Part model, mm, in its own coordinate system. A direction names the side the tool comes from. Round coordinates to 2 decimals unless told otherwise and drop trailing zeros. Write each loop counter-clockwise with the first axis right and the second up, starting at its lowest first coordinate (ties: lowest second). Pieces come first, ordered by that corner, then holes. Notation, with made-up numbers: M -9,23.25 L 2,23.25 A7 ccw 2,30.25 Z; hole C 37.25,-10 d3. An arc over 180 degrees is marked long. Answer as a JSON object with one key per item and string values. Group by question number.
1. Drop flat-ended pins along their axis: pin 1 (2 mm diameter, centred on x = 2.5, z = 1.5, fed in from -Y); pin 2 (1 mm diameter, centred on x = -7, z = 0.5, fed in from -Y); pin 3 (3 mm diameter, centred on y = 6, z = 0.5, fed in from -X). Give the stop position or say it passes through.
2. Band-saw the part on D-D, the plane x = -11.5. Write the cut outline in (y, z).
3. Band-saw the part on A-A, the plane y = 0. Write the cut outline in (x, z).
4. Two-plate mould, pull along X, no slides. Class faces 1 (the face through (-11.99, 0.53, -3.25)), 2 (the face through (-3.6, 14.3, -3.5)), 3 (the face through (-3.47, -15.62, 0.05)): +X half, -X half, draft (parallel to the pull), parting line (faces both ways), or undercut.
5. Band-saw the part on C-C, the plane z = -1.75. Write the cut outline in (x, y), plus the area to 3 significant figures.
6. Drill centre lines: line 1 (Y direction, x = 0, z = -3.15); line 2 (Y direction, x = 0, z = -1.25); line 3 (Z direction, x = -8.5, y = -11.5). Where is each one in solid material? Low to high. Write a range as from..to.
7. Which spindle directions (+Z, -Z, +X, -X, +Y, -Y) get a long thin tool onto all of the face, cutting with end or side? Do faces 4 (the face through (-11.99, 0.53, 3.25)), 5 (the face through (2, 12, -3)), 6 (the face through (-2.17, -9.76, -0.05)). Say none if no direction does.
from build123d import *

# Parameters (mm, degrees)
SKETCH_R      = 16
SKETCH_R_2    = 14.5
PAD_DEPTH     = 3.5
SKETCH001_R   = 14.5
SKETCH001_R_2 = 12
PAD001_DEPTH  = 3
SKETCH002_R   = 12
SKETCH002_R_2 = 10
PAD002_DEPTH  = 3.5


with BuildPart() as part:
    # Sketch → Pad (new body, symmetric)
    with BuildSketch(Plane.XY):
        Circle(SKETCH_R)
        Circle(SKETCH_R_2, mode=Mode.SUBTRACT)
    extrude(amount=PAD_DEPTH, both=True)

    # Sketch001 → Pad001 (join, symmetric)
    with BuildSketch(Plane.XY):
        Circle(SKETCH001_R)
        Circle(SKETCH001_R_2, mode=Mode.SUBTRACT)
    extrude(amount=PAD001_DEPTH, both=True)

    # Sketch002 → Pad002 (join, symmetric)
    with BuildSketch(Plane.XY):
        Circle(SKETCH002_R)
        Circle(SKETCH002_R_2, mode=Mode.SUBTRACT)
    extrude(amount=PAD002_DEPTH, both=True)


solid = part.part
Worked answers:
{
 "1": {"pin 1": "stops at y = -15.93", "pin 2": "stops at y = -14.62", "pin 3": "stops at x = -15.35"},
 "2": {"outline": "M -11.12,-3.5 L -8.83,-3.5 L -8.83,-3 L -3.43,-3 L -3.43,-3.5 L 3.43,-3.5 L 3.43,-3 L 8.83,-3 L 8.83,-3.5 L 11.12,-3.5 L 11.12,3.5 L 8.83,3.5 L 8.83,3 L 3.43,3 L 3.43,3.5 L -3.43,3.5 L -3.43,3 L -8.83,3 L -8.83,3.5 L -11.12,3.5 Z"},
 "3": {"outline": "M -16,-3.5 L -14.5,-3.5 L -14.5,-3 L -12,-3 L -12,-3.5 L -10,-3.5 L -10,3.5 L -12,3.5 L -12,3 L -14.5,3 L -14.5,3.5 L -16,3.5 Z; M 10,-3.5 L 12,-3.5 L 12,-3 L 14.5,-3 L 14.5,-3.5 L 16,-3.5 L 16,3.5 L 14.5,3.5 L 14.5,3 L 12,3 L 12,3.5 L 10,3.5 Z"},
 "4": {"face 1": "undercut", "face 2": "draft", "face 3": "parting line"},
 "5": {"outline": "C 0,0 d32; hole C 0,0 d20", "area": "490 mm^2"},
 "6": {"line 1": "y = -16..-14.5, -12..-10, 10..12, 14.5..16", "line 2": "y = -16..-10, 10..16", "line 3": "z = -3..3"},
 "7": {"face 4": "+Z", "face 5": "-Z", "face 6": "+Z, -Z"}
}
